Geometry: see drawing. Coordinates: mm, zero at the bounding-box minimum. A direction names the side the tool comes from. Round coordinates to 2 decimals unless told otherwise and drop trailing zeros. Loops run counter-clockwise (first coordinate to the right, second up) from the corner with the lowest first, then second, coordinate; pieces in that order, holes last. Notation, with made-up numbers: (3, -0.5) -> (39, -0.5) arc R14 ccw to (39, 5.5) -> close; hole circle Ø8 at (13, 88.25). An arc over 180 degrees is marked (long way). Answer in a Markdown table with one row per item.
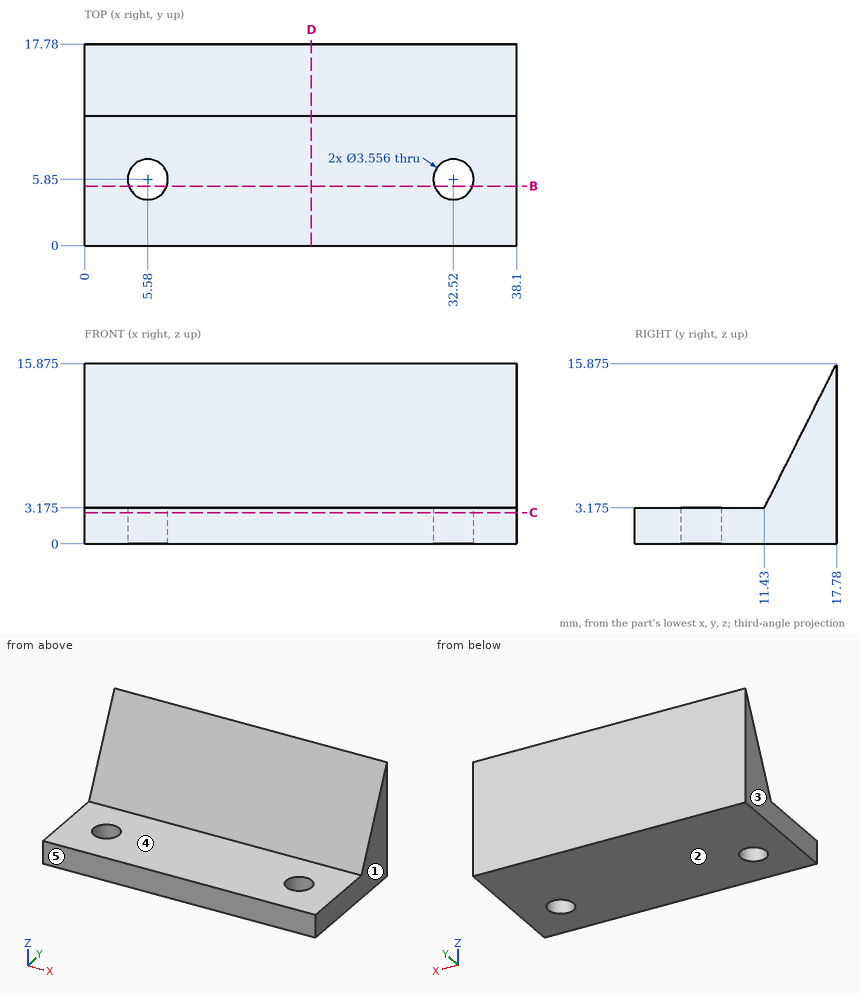
Item 1: Mould query, pull axis X, two halves, no side actions, for the marked faces 1, 2 and 3. Classes: released by +X, released by -X, zero draft, split by the parting line, or undercut.
Ans:
| item | result |
|---|---|
| face 1 | released by +X |
| face 2 | zero draft |
| face 3 | released by -X |
Item 2: Set-up query: the marked faces 4 and 5. Return all of +Z, -Z, +X, -X, +Y, -Y with unobstructed straight access to the full face (end or side cutting, diameter ignored); none if empty.
Ans:
| item | result |
|---|---|
| face 4 | +Z, +X, -X, -Y |
| face 5 | +Z, -Z, +X, -X, -Y |
Item 3: Section query C-C, the plane z = 2.75. Output: boundary loops of the cut face in (x, y).
Ans:
| item | result |
|---|---|
| outline | (0, 0) -> (38.1, 0) -> (38.1, 17.78) -> (0, 17.78) -> close; hole circle Ø3.56 at (5.58, 5.85); hole circle Ø3.56 at (32.52, 5.85) |
Item 4: Ray query, L1, parallel to Z at x = 30, y = 4.5 (1 decimal); L2, parallel to Y at x = 5, z = 7.5; L3, parallel to Z at x = 31, y = 14 (1 decimal). Return the intervals inside material, ascending.
Ans:
| item | result |
|---|---|
| L1 | 0 to 3.2 |
| L2 | 13.59 to 17.78 |
| L3 | 0 to 8.3 |
Item 5: Section query D-D, the plane x = 20. Output: boundary loops of the cut face in (y, z) (1 decimal).
Ans:
| item | result |
|---|---|
| outline | (0, 0) -> (17.8, 0) -> (17.8, 15.9) -> (11.4, 3.2) -> (0, 3.2) -> close |
Item 6: Section query B-B, the plane y = 5.25. Output: boundary loops of the cut face in (x, z) (1 decimal).
Ans:
| item | result |
|---|---|
| outline | (0, 0) -> (3.9, 0) -> (3.9, 3.2) -> (0, 3.2) -> close; (7.3, 0) -> (30.8, 0) -> (30.8, 3.2) -> (7.3, 3.2) -> close; (34.2, 0) -> (38.1, 0) -> (38.1, 3.2) -> (34.2, 3.2) -> close |
